Input: dimensioned drawing with shaded views. Units: mm. Origin: part minimum x, y, z. A direction names the side the tool comes from. Round coordinates to 2 decimals unless told otherwise and drop trailing zeros. Write each loop counter-clockwise with the first axis right and the second up, starting at its lowest first coordinate (ties: lowest second). Pieces come first, ordered by that corner, then holes. Notation, with made-up numbers: M 14,-5.75 L 38,-5.75 A26 ccw 38,12.25 Z; hole C 48.5,46.25 d6. An arc over 180 degrees is marked long. Answer as CSV lines item,"result". Start each with the question number.
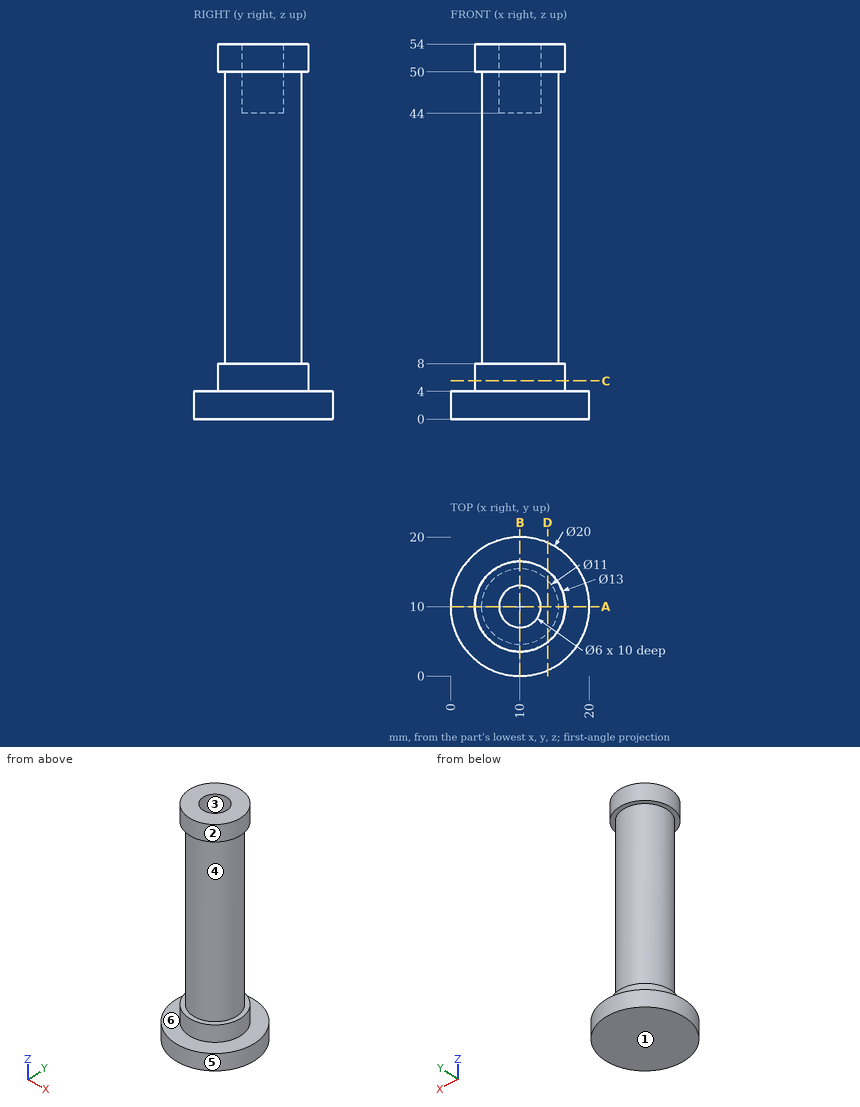
Item 1: Pin query (flat end, axial travel): pin 1 Ø5 at (x, z) = (15.5, 8) entering from +Y; pin 2 Ø1.8 at (x, y) = (11, 8.5) entering from +Z; pin 3 Ø4 at (x, z) = (3.5, 14) entering from -Y; pin 4 Ø2 at (y, z) = (17.5, 13.5) entering from +X. Return the tip coordinate at first contact, or that it passes through.
Item 2: Line query: line 1 (Y direction, x = 10, z = 47); line 2 (Z direction, x = 14, y = 14.5); line 3 (Z direction, x = 7, y = 16.5). Output: solid intervals per line, ascending. Write a range as [from, to].
Item 3: Cut plane A-A, the plane y = 10. Return loops of the section in (x, z), plus the area to 3 significant figures.
Item 4: Cut plane D-D, the plane x = 14. Return loops of the section in (y, z).
Item 5: Cut plane C-C, the plane z = 5.5. Return loops of the section in (x, y).
Item 6: Access query for the marked faces 4, 5 and 6. Directions: +Z, -Z, +X, -X, +Y, -Y. A direction counts if a zero-diameter tool reaches every point of the face in a straight line with its end or side. Return the directions, or none.
Item 7: Draft query along Y for the marked faces 1, 2 and 3. Return one class per face: +Y half, -Y half, draft (parallel to the pull), parting line (faces both ways), or undercut.
Results list:
1,pin 1,"y = 15.77"
1,pin 2,"z = 44"
1,pin 3,"y = 6.84"
1,pin 4,"through"
2,line 1,"[4.5, 7], [13, 15.5]"
2,line 2,"[0, 8], [50, 54]"
2,line 3,"[0, 4]"
3,outline,"M 0,0 L 20,0 L 20,4 L 16.5,4 L 16.5,8 L 15.5,8 L 15.5,50 L 16.5,50 L 16.5,54 L 13,54 L 13,44 L 7,44 L 7,54 L 3.5,54 L 3.5,50 L 4.5,50 L 4.5,8 L 3.5,8 L 3.5,4 L 0,4 Z"
3,area,"586 mm²"
4,outline,"M 0.83,0 L 19.17,0 L 19.17,4 L 15.12,4 L 15.12,8 L 13.77,8 L 13.77,50 L 15.12,50 L 15.12,54 L 4.88,54 L 4.88,50 L 6.23,50 L 6.23,8 L 4.88,8 L 4.88,4 L 0.83,4 Z"
5,outline,"C 10,10 d13"
6,face 4,"none"
6,face 5,"+Z, -Z"
6,face 6,"+Z"
7,face 1,"draft"
7,face 2,"parting line"
7,face 3,"undercut"
